from build123d import *

# Parameters (mm, degrees)
SKETCH1_W                                        = 114.3
SKETCH1_H                                        = 114.3
STOCK_DEPTH                                      = 8.255
CBORE_FOR_1_4_SOCKET_HEAD_CAP_SCREW1_D           = 6.7564
CBORE_FOR_1_4_SOCKET_HEAD_CAP_SCREW1_CBORE_D     = 11.1125
CBORE_FOR_1_4_SOCKET_HEAD_CAP_SCREW1_CBORE_DEPTH = 6.35
F_5_32_0_15625_DIAMETER_HOLE1_D                  = 3.96875
CBORE_FOR_4_SOCKET_HEAD_CAP_SCREW1_D             = 3.2639
CBORE_FOR_4_SOCKET_HEAD_CAP_SCREW1_DEPTH         = 8.255
CBORE_FOR_4_SOCKET_HEAD_CAP_SCREW1_CBORE_D       = 5.55752
CBORE_FOR_4_SOCKET_HEAD_CAP_SCREW1_CBORE_DEPTH   = 2.8448
F_1_4_20_TAPPED_HOLE1_D                          = 5.1054


with BuildPart() as part:
    # Sketch1 → stock (new body)
    with BuildSketch(Plane(origin=(0, 0, 0), x_dir=(1, 0, 0), z_dir=(0, 1, 0))):
        Rectangle(SKETCH1_W, SKETCH1_H)
    extrude(amount=STOCK_DEPTH)

    # CBORE for 1/4 Socket Head Cap Screw1 (through all)
    with Locations(Plane(origin=(0, 0, 0), x_dir=(-1, 0, 0), z_dir=(0, -1, 0))):
        with Locations((0, 0)):
            CounterBoreHole(CBORE_FOR_1_4_SOCKET_HEAD_CAP_SCREW1_D / 2, CBORE_FOR_1_4_SOCKET_HEAD_CAP_SCREW1_CBORE_D / 2, CBORE_FOR_1_4_SOCKET_HEAD_CAP_SCREW1_CBORE_DEPTH)

    # 5/32 (0.15625) Diameter Hole1 (through all)
    with Locations(Plane(origin=(0, 8.255, 0), x_dir=(1, 0, 0), z_dir=(0, 1, 0))):
        with Locations((44.45, 0), (-44.45, 0)):
            Hole(F_5_32_0_15625_DIAMETER_HOLE1_D / 2)

    # CBORE for #4 Socket Head Cap Screw1
    with Locations(Plane(origin=(0, 0, 0), x_dir=(-1, 0, 0), z_dir=(0, -1, 0))):
        with Locations((44.45, -44.45), (44.45, 44.45), (-44.45, 44.45), (-44.45, -44.45), (0, 0)):
            CounterBoreHole(CBORE_FOR_4_SOCKET_HEAD_CAP_SCREW1_D / 2, CBORE_FOR_4_SOCKET_HEAD_CAP_SCREW1_CBORE_D / 2, CBORE_FOR_4_SOCKET_HEAD_CAP_SCREW1_CBORE_DEPTH, depth=CBORE_FOR_4_SOCKET_HEAD_CAP_SCREW1_DEPTH)

    # 1/4-20 Tapped Hole1 (through all)
    with Locations(Plane(origin=(0, 0, 0), x_dir=(-1, 0, 0), z_dir=(0, -1, 0))):
        with Locations((50.8, -38.1), (25.4, -38.1), (25.4, 0), (50.8, 0), (50.8, 38.1), (25.4, 38.1), (-25.4, 38.1), (-50.8, 38.1), (-50.8, 0), (-25.4, 0), (-25.4, -38.1), (-50.8, -38.1)):
            Hole(F_1_4_20_TAPPED_HOLE1_D / 2)


solid = part.part
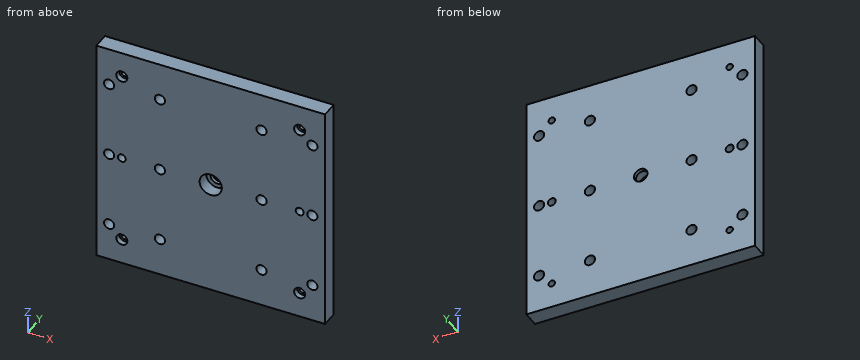
Read the model definition and answer for the solid it produces. Units are mm, in the model's axes. Round coordinates to 2 decimals unless told otherwise and drop trailing zeros. Write each loop counter-clockwise with the first axis right and the second up, starting at its lowest first coordinate (ties: lowest second). Pieces come first, ordered by that corner, then holes.
1. The part is cut by section A-A, the plane x = 25.4. Determine the outline of the cut face in (y, z) (3 decimals), then the cut area to 3 significant figures.
2. Given pin 1 Ø4.5 at (x, z) = (25.4, -38.1) entering from +Y; pin 2 Ø1.7 at (x, z) = (45.5, -45) entering from -Y; pin 3 Ø9 at (x, z) = (0, 0) entering from -Y, each flat-ended and moving along its own axis, determine where each tip first touches the part or whether it passes through.
3. Straight lines are drawn through the part: L1, parallel to X at y = 5, z = 38.1; L2, parallel to Z at x = 51, y = 1.5; L3, parallel to Z at x = -50.8, y = 1.75. For each, find the intervals that lie inside material, in ascending order.
4. The part is cut by section C-C, the plane x = 0. Determine the outline of the cut face in (y, z) (3 decimals).
5. The part is cut by section D-D, the plane z = -38.1. Determine the outline of the cut face in (x, y) (3 decimals), then the cut area to 3 significant figures.
6. The part is cut by section B-B, the plane z = 44.45. Determine the outline of the cut face in (x, y) (3 decimals).
Values:
1. outline: (0, -57.15) - (8.255, -57.15) - (8.255, -40.653) - (0, -40.653) - close; (0, -35.547) - (8.255, -35.547) - (8.255, -2.553) - (0, -2.553) - close; (0, 2.553) - (8.255, 2.553) - (8.255, 35.547) - (0, 35.547) - close; (0, 40.653) - (8.255, 40.653) - (8.255, 57.15) - (0, 57.15) - close
1. area: 817 mm2
2. pin 1: passes through
2. pin 2: stops at y = 2.84
2. pin 3: stops at y = 6.35
3. L1: x = -57.15 to -53.35, -48.25 to -27.95, -22.85 to 22.85, 27.95 to 48.25, 53.35 to 57.15
3. L2: z = -57.15 to -40.64, -35.56 to -2.54, 2.54 to 35.56, 40.64 to 57.15
3. L3: z = -57.15 to -40.65, -35.55 to -2.55, 2.55 to 35.55, 40.65 to 57.15
4. outline: (0, -57.15) - (8.255, -57.15) - (8.255, -3.378) - (6.35, -3.378) - (6.35, -5.556) - (0, -5.556) - close; (0, 5.556) - (6.35, 5.556) - (6.35, 3.378) - (8.255, 3.378) - (8.255, 57.15) - (0, 57.15) - close
5. outline: (-57.15, 0) - (-53.353, 0) - (-53.353, 8.255) - (-57.15, 8.255) - close; (-48.247, 0) - (-27.953, 0) - (-27.953, 8.255) - (-48.247, 8.255) - close; (-22.847, 0) - (22.847, 0) - (22.847, 8.255) - (-22.847, 8.255) - close; (27.953, 0) - (48.247, 0) - (48.247, 8.255) - (27.953, 8.255) - close; (53.353, 0) - (57.15, 0) - (57.15, 8.255) - (53.353, 8.255) - close
5. area: 775 mm2
6. outline: (-57.15, 0) - (-47.229, 0) - (-47.229, 2.845) - (-46.082, 2.845) - (-46.082, 8.255) - (-57.15, 8.255) - close; (-42.818, 2.845) - (-41.671, 2.845) - (-41.671, 0) - (41.671, 0) - (41.671, 2.845) - (42.818, 2.845) - (42.818, 8.255) - (-42.818, 8.255) - close; (46.082, 2.845) - (47.229, 2.845) - (47.229, 0) - (57.15, 0) - (57.15, 8.255) - (46.082, 8.255) - close
